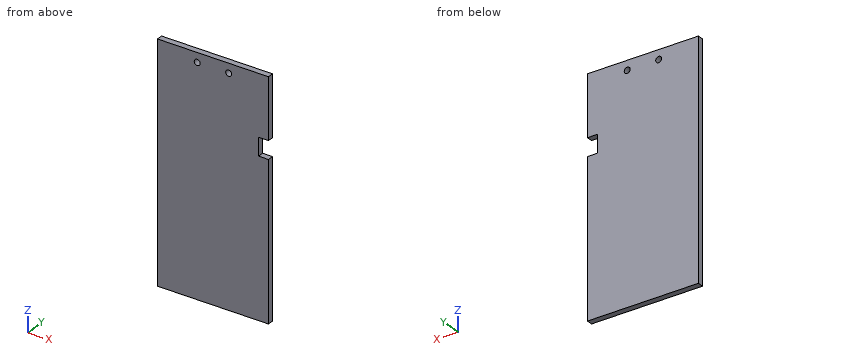
```python
from build123d import *

# Parameters (mm, degrees)
SKETCH1_W             = 56
SKETCH1_H             = 98
BOSS_EXTRUDE1_DEPTH   = 3
SKETCH4_W             = 56
SKETCH4_H             = 3
BOSS_EXTRUDE3_DEPTH   = 20
SKETCH9_W             = 5
SKETCH9_H             = 9
CUT_EXTRUDE1_DEPTH    = 10
CROQUIS1_R            = 1.5
CORTAR_EXTRUIR1_DEPTH = 10


with BuildPart() as part:
    # Sketch1 → Boss-Extrude1 (new body)
    with BuildSketch(Plane(origin=(0, 0, 0), x_dir=(1, 0, 0), z_dir=(0, 1, 0))):
        with Locations((28, 49)):
            Rectangle(SKETCH1_W, SKETCH1_H)
    extrude(amount=BOSS_EXTRUDE1_DEPTH)

    # Sketch4 → Boss-Extrude3 (add)
    with BuildSketch(Plane.XY):
        with Locations((28, 1.5)):
            Rectangle(SKETCH4_W, SKETCH4_H)
    extrude(amount=BOSS_EXTRUDE3_DEPTH)

    # Sketch9 → Cut-Extrude1 (cut)
    with BuildSketch(Plane(origin=(0, 3, 0), x_dir=(1, 0, 0), z_dir=(0, 1, 0))):
        with Locations((53.5, 15)):
            Rectangle(SKETCH9_W, SKETCH9_H)
    extrude(amount=-CUT_EXTRUDE1_DEPTH, mode=Mode.SUBTRACT)

    # Croquis1 → Cortar-Extruir1 (cut)
    with BuildSketch(Plane(origin=(0, 3, 0), x_dir=(1, 0, 0), z_dir=(0, 1, 0))):
        with Locations(Location((20.06, -15.24, 0), (0, 0, 270))):
            Circle(CROQUIS1_R)
        with Locations(Location((35.94, -15.24, 0), (0, 0, 90))):
            Circle(CROQUIS1_R)
    extrude(amount=-CORTAR_EXTRUIR1_DEPTH, mode=Mode.SUBTRACT)


solid = part.part
```
Read the model definition and answer for the solid it produces. Units are mm, in the model's axes. Coordinates: 2 decimals unless noted, no trailing zeros. Order: outer loops, then holes, each group sorted by start corner. A loop starts at its lowest first (then second) coordinate and runs counter-clockwise, first axis right, second up. Notation, with made-up numbers: (13, 88) - (26, 88) arc R15 ccw to (26, 94) - close; hole circle Ø10 at (85.5, -15). An arc over 180 degrees is marked (long way). Answer as a JSON object with one key per item and string values. Group by question number.
Item 1: Section B-B (z = 15.24) is taken. Give the vertices of the cut face in (x, y).
Item 2: Consider probe 1 along X at (y, z) = (1.8, 15.24); probe 2 along Z at (x, y) = (20, 0.45); probe 3 along X at (y, z) = (2.5, -13). Determine where each line is inside the solid, lowest interval first. Write a range as from..to.
Item 3: A flat-ended cylindrical pin translates along its axis: P1, Ø3, axis at x = 34.5, z = -83, coming from the -Y side. Find the tip coordinate at first contact, or state that the pin passes through.
Item 4: Section A-A (x = 35.94) is taken. Give the vertices of the cut face in (y, z).
Results are:
{
 "1": {"outline": "(0, 0) - (18.56, 0) - (18.56, 3) - (0, 3) - close; (21.56, 0) - (34.44, 0) - (34.44, 3) - (21.56, 3) - close; (37.44, 0) - (56, 0) - (56, 3) - (37.44, 3) - close"},
 "2": {"probe 1": "x = 0..18.56, 21.56..34.44, 37.44..56", "probe 2": "z = -98..13.74, 16.74..20", "probe 3": "x = 0..51"},
 "3": {"P1": "stops at y = 0"},
 "4": {"outline": "(0, -98) - (3, -98) - (3, 13.74) - (0, 13.74) - close; (0, 16.74) - (3, 16.74) - (3, 20) - (0, 20) - close"}
}
